Can you work these out from the model? Positions are in its coordinate system, mm. A direction names the side the tool comes from. Give positions to 0.01 mm unless a question says otherwise; leave off trailing zeros. Loops run counter-clockwise (first coordinate to the right, second up) from the corner with the lowest first, then second, coordinate; pieces in that order, holes last. Notation, with made-up numbers: (73, 45) - (115, 45) arc R15 ccw to (115, 59) - close; hole circle Ø8 at (-25.75, 21). An arc over 180 degrees is marked (long way). Answer as a JSON object with one key per item and string values. Group by question number.
Item 1: Please list where these lines run through material, in increasing order: L1, parallel to Z at x = 0, y = -6; L2, parallel to X at y = -18.75, z = -3; L3, parallel to X at y = -14.25, z = -4.
Item 2: Will these pins go through, and if not, where does the flat tip stop? pin 1 (1.5 mm diameter, centred on y = -2.5, z = -97.5, fed in from -X); pin 2 (4 mm diameter, centred on y = -15, z = 22, fed in from +X); pin 3 (3 mm diameter, centred on x = 110.5, y = -15.5, fed in from -Z).
Item 3: Suppose I cut it at B-B on y = -3.75. Write out the boundary of the cut face in (x, z).
Item 4: Suppose I cut it at C-C on x = -118.5. Write out the boundary of the cut face in (y, z).
Item 5: Which directions (+Z, -Z, +X, -X, +Y, -Y) give clear straight access to the entire face, cutting with the end or side of a thin tool? Please do faces 1 (the flat face through (88.413, -12.522, -47.266)), 2 (the flat face through (-99, -13, -21.532)), 3 (the cylindrical face through (132.734, -12.878, 84.814)).
Item 6: Suppose I cut it at D-D on z = 33. Write out the boundary of the cut face in (x, y), and give its area (3 significant figures).
Item 7: Thinking about a two-plate mould opening in X: for faces 4 (the flat face through (91.261, -12.522, 37.135)), 5 (the flat face through (-95, -13, 29.268)), 6 (the cylindrical face through (-17.89, -12.88, -13.72)), which applies, pulls with the +X half, pulls with the -X half, needs draft (parallel to the pull), parting line crosses it, or undercut?
Item 8: Suppose I cut it at A-A on x = -10.5. Write out the boundary of the cut face in (y, z), and give its area (3 significant figures).
from build123d import *

# Parameters (mm, degrees)
F1_DEPTH  = 25.4
F2_R      = 22.5453784596
F3_DEPTH  = 25.401
F4_R      = 15.5169822629
F4_R_2    = 14.6151483758
F4_R_3    = 13.5851891759
F5_DEPTH  = 419
F6_R      = 14.3828522328
F7_DEPTH  = 25.401
F8_R      = 13.6217726984
F9_DEPTH  = 25.4
F10_R     = 13.3826357349
F11_DEPTH = 25.4


# Not quite as in the source:
# - an extrude ends at something that could not be found from the text; its depth is read off the source's solid


with BuildPart() as f1:
    # F0 (on Front) → F1 (new body)
    with BuildSketch(Plane.XZ):
        with BuildLine():
            ThreePointArc((50.3233435561, -12.5877974986), (51.4847298632, -6.3414622483), (51.873804107, 0))
            ThreePointArc((51.873804107, 0), (51.7629612184, 3.3893064834), (51.4309062461, 6.7641285647))
            ThreePointArc((51.4309062461, 6.7641285647), (42.7546046022, 29.3757610599), (24.7585971482, 45.5840259278))
            ThreePointArc((24.7585971482, 45.5840259278), (-12.1730496974, 50.4252755431), (-42.8284505735, 29.2679923125))
            ThreePointArc((-42.8284505735, 29.2679923125), (-51.683323237, 4.4413569672), (-47.1939000029, -21.5320076875))
            ThreePointArc((-47.1939000029, -21.5320076875), (-18.7719046051, -48.3581135905), (20.3057196076, -47.7343618764))
            ThreePointArc((20.3057196076, -47.7343618764), (39.4453595209, -33.6890956364), (50.3233435561, -12.5877974986))
        make_face()
        with BuildLine():
            ThreePointArc((24.7585971482, 45.5840259278), (42.7546046022, 29.3757610599), (51.4309062461, 6.7641285647))
            Line((51.4309062461, 6.7641285647), (132.2230654066, 68.3692177878))
            ThreePointArc((132.2230654066, 68.3692177878), (140.3155469651, 104.8046621717), (103.3515533001, 109.9711926872))
            Line((103.3515533001, 109.9711926872), (24.7585971482, 45.5840259278))
        make_face()
        with BuildLine():
            Line((125.4517560768, -80.9857626154), (50.3233435561, -12.5877974986))
            ThreePointArc((50.3233435561, -12.5877974986), (39.4453595209, -33.6890956364), (20.3057196076, -47.7343618764))
            Line((20.3057196076, -47.7343618764), (93.0013113713, -118.7126045859))
            ThreePointArc((93.0013113713, -118.7126045859), (127.5656184462, -115.6234022642), (125.4517560768, -80.9857626154))
        make_face()
        with BuildLine():
            ThreePointArc((-47.1939000029, -21.5320076875), (-51.683323237, 4.4413569672), (-42.8284505735, 29.2679923125))
            Line((-42.8284505735, 29.2679923125), (-148.7939000029, 29.2679923125))
            ThreePointArc((-148.7939000029, 29.2679923125), (-174.1939000029, 3.8679923125), (-148.7939000029, -21.5320076875))
            Line((-148.7939000029, -21.5320076875), (-47.1939000029, -21.5320076875))
        make_face()
    extrude(amount=F1_DEPTH)

    # F2 (on face) → F3 (cut, through all)
    with BuildSketch(Plane.XZ.offset(25.4)):
        Circle(F2_R)
    extrude(amount=-F3_DEPTH, mode=Mode.SUBTRACT)

    # F4 (on face) → F5 (cut, through all)
    with BuildSketch(Plane.XZ.offset(25.4)):
        with Locations((119.4483449899, 90.3229536493)):
            Circle(F4_R)
        with Locations((108.694701762, -99.3917325452)):
            Circle(F4_R_2)
        with Locations((-148.7939000029, 3.8679923125)):
            Circle(F4_R_3)
    extrude(amount=F5_DEPTH, mode=Mode.SUBTRACT)

    # F6 (on face) → F7 (cut, through all)
    with BuildSketch(Plane.XZ.offset(25.4)):
        with Locations((119.4483449899, 90.3229536493)):
            Circle(F6_R)
    extrude(amount=-F7_DEPTH, mode=Mode.SUBTRACT)

    # F8 (on face) → F9 (cut)
    with BuildSketch(Plane.XZ.offset(25.4)):
        with Locations((108.694701762, -99.3917325452)):
            Circle(F8_R)
    extrude(amount=-F9_DEPTH, mode=Mode.SUBTRACT)

    # F10 (on face) → F11 (cut)
    with BuildSketch(Plane.XZ.offset(25.4)):
        with Locations((-148.7939000029, 3.8679923125)):
            Circle(F10_R)
    extrude(amount=-F11_DEPTH, mode=Mode.SUBTRACT)


solid = f1.part
Worked out:
{
 "1": {"L1": "z = -51.87 to -22.55, 22.55 to 51.87", "L2": "x = -173.25 to -160.28, -137.31 to -22.34, 22.34 to 51.79", "L3": "x = -172.94 to -159.62, -137.97 to -22.19, 22.19 to 51.72"},
 "2": {"pin 1": "stops at x = 70.51", "pin 2": "stops at x = 74.03", "pin 3": "stops at z = -124.28"},
 "3": {"outline": "(-148.79, -21.53) - (-47.19, -21.53) arc R51.87 ccw to (20.31, -47.73) - (93, -118.71) arc R24.89 ccw to (125.45, -80.99) - (50.32, -12.59) arc R51.87 ccw to (51.43, 6.76) - (132.22, 68.37) arc R25.4 ccw (long way) to (103.35, 109.97) - (24.76, 45.58) arc R51.87 ccw to (-42.83, 29.27) - (-148.79, 29.27) arc R25.4 ccw to start; hole circle Ø26.77 at (-148.79, 3.87); hole circle Ø45.09 at (0, 0); hole circle Ø27.24 at (108.69, -99.39); hole circle Ø28.77 at (119.45, 90.32)"},
 "4": {"outline": "(-25.4, -21.53) - (0, -21.53) - (0, 29.27) - (-25.4, 29.27) - close"},
 "5": {"face 1": "+X, +Y, -Y", "face 2": "-Z, -X, +Y, -Y", "face 3": "+Y, -Y"},
 "6": {"outline": "(-40.02, -25.4) - (85.84, -25.4) - (85.84, 0) - (-40.02, 0) - close", "area": "3,200 mm2"},
 "7": {"face 4": "pulls with the +X half", "face 5": "needs draft", "face 6": "undercut"},
 "8": {"outline": "(-25.4, -50.8) - (0, -50.8) - (0, -19.95) - (-25.4, -19.95) - close; (-25.4, 19.95) - (0, 19.95) - (0, 50.8) - (-25.4, 50.8) - close", "area": "1,570 mm2"}
}
